from build123d import *

# Parameters (mm, degrees)
F1_DEPTH = 127
F3_DEPTH = 1.00176


with BuildPart() as f1:
    # F0 (on Front) → F1 (new body, symmetric)
    with BuildSketch(Plane.XZ):
        with BuildLine():
            ThreePointArc((-13.5001, 1.99898), (-12.9146123135, 0.5854876865), (-11.50112, 0))
            Line((-11.50112, 0), (11.50112, 0))
            ThreePointArc((11.50112, 0), (12.9146123135, 0.5854876865), (13.5001, 1.99898))
            Line((13.5001, 1.99898), (13.5001, 5.4991))
            ThreePointArc((13.5001, 5.4991), (13.7932158177, 6.2067441823), (14.50086, 6.49986))
            Line((14.50086, 6.49986), (18.3281093243, 6.49986))
            Line((18.3281093243, 6.49986), (18.3281093243, 7.50062))
            Line((18.3281093243, 7.50062), (14.5161, 7.50062))
            ThreePointArc((14.5161, 7.50062), (13.1026076865, 6.9151323135), (12.51712, 5.50164))
            Line((12.51712, 5.50164), (12.51712, 2.00152))
            ThreePointArc((12.51712, 2.00152), (12.2240041823, 1.2938758177), (11.51636, 1.00076))
            Line((11.51636, 1.00076), (-11.48334, 1.00076))
            ThreePointArc((-11.48334, 1.00076), (-12.1909841823, 1.2938758177), (-12.4841, 2.00152))
            Line((-12.4841, 2.00152), (-12.4841, 5.50164))
            ThreePointArc((-12.4841, 5.50164), (-13.0695876865, 6.9151323135), (-14.48308, 7.50062))
            Line((-14.48308, 7.50062), (-16.6730906757, 7.50062))
            Line((-16.6730906757, 7.50062), (-16.6730906757, 6.49986))
            Line((-16.6730906757, 6.49986), (-14.50086, 6.49986))
            ThreePointArc((-14.50086, 6.49986), (-13.7932158177, 6.2067441823), (-13.5001, 5.4991))
            Line((-13.5001, 5.4991), (-13.5001, 1.99898))
        make_face()
    extrude(amount=F1_DEPTH, both=True)

    # F2 (on face) → F3 (cut, through all)
    with BuildSketch(Plane.XY.offset(1.00076)):
        with BuildLine():
            ThreePointArc((2.59969, 9.89965), (0, 12.49934), (-2.59969, 9.89965))
            Line((-2.59969, 9.89965), (-2.59969, -9.89965))
            ThreePointArc((-2.59969, -9.89965), (0, -12.49934), (2.59969, -9.89965))
            Line((2.59969, -9.89965), (2.59969, 9.89965))
        make_face()
        with BuildLine():
            ThreePointArc((-2.59969, 26.09977), (0, 23.50008), (2.59969, 26.09977))
            Line((2.59969, 26.09977), (2.59969, 45.89907))
            ThreePointArc((2.59969, 45.89907), (0, 48.49876), (-2.59969, 45.89907))
            Line((-2.59969, 45.89907), (-2.59969, 26.09977))
        make_face()
        with BuildLine():
            ThreePointArc((-2.59969, 62.09919), (0, 59.4995), (2.59969, 62.09919))
            Line((2.59969, 62.09919), (2.59969, 81.89849))
            ThreePointArc((2.59969, 81.89849), (0, 84.49818), (-2.59969, 81.89849))
            Line((-2.59969, 81.89849), (-2.59969, 62.09919))
        make_face()
        with BuildLine():
            ThreePointArc((-2.59969, 98.09861), (0, 95.49892), (2.59969, 98.09861))
            Line((2.59969, 98.09861), (2.59969, 117.89791))
            ThreePointArc((2.59969, 117.89791), (0, 120.4976), (-2.59969, 117.89791))
            Line((-2.59969, 117.89791), (-2.59969, 98.09861))
        make_face()
        with BuildLine():
            ThreePointArc((-2.59969, -45.89907), (0, -48.49876), (2.59969, -45.89907))
            Line((2.59969, -45.89907), (2.59969, -26.09977))
            ThreePointArc((2.59969, -26.09977), (0, -23.50008), (-2.59969, -26.09977))
            Line((-2.59969, -26.09977), (-2.59969, -45.89907))
        make_face()
        with BuildLine():
            ThreePointArc((-2.59969, -81.89849), (0, -84.49818), (2.59969, -81.89849))
            Line((2.59969, -81.89849), (2.59969, -62.09919))
            ThreePointArc((2.59969, -62.09919), (0, -59.4995), (-2.59969, -62.09919))
            Line((-2.59969, -62.09919), (-2.59969, -81.89849))
        make_face()
        with BuildLine():
            ThreePointArc((-2.59969, -117.89791), (0, -120.4976), (2.59969, -117.89791))
            Line((2.59969, -117.89791), (2.59969, -98.09861))
            ThreePointArc((2.59969, -98.09861), (0, -95.49892), (-2.59969, -98.09861))
            Line((-2.59969, -98.09861), (-2.59969, -117.89791))
        make_face()
    extrude(amount=-F3_DEPTH, mode=Mode.SUBTRACT)


solid = f1.part
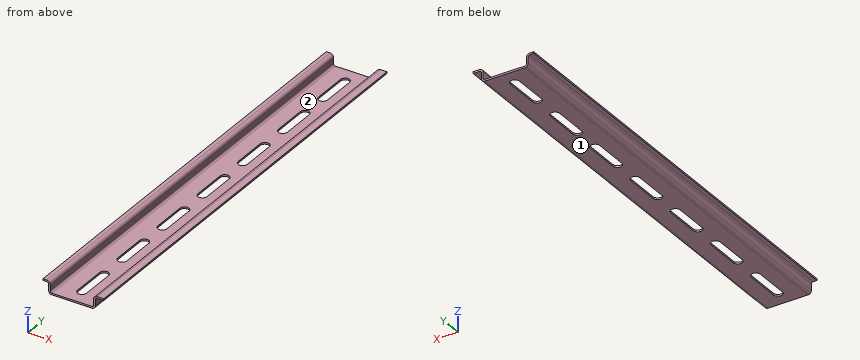
Source: CAD feature listing. Evaluate the final solid. Frame: model axes, mm. Face numbers are marked on the shaded views. Coordinates: 2 decimals unless noted, no trailing zeros. Order: outer loops, then holes, each group sorted by start corner. A loop starts at its lowest first (then second) coordinate and runs counter-clockwise, first axis right, second up.
Item 1: Material intervals for line 1 (X direction, y = -48.5, z = 3); line 2 (Z direction, x = -4.5, y = 21.5); line 3 (Z direction, x = 15, y = -31.5), sorted ascending.
Output values:
line 1: x = -13.5 to -12.48, 12.52 to 13.5
line 2: z = 0 to 1
line 3: z = 6.5 to 7.5
Item 2: Cut plane B-B (z = 3.25). Return loops of the section in (x, y), plus the area to 3 significant figures.
Output values:
outline: (-13.5, -127) - (-12.48, -127) - (-12.48, 127) - (-13.5, 127) - close; (12.52, -127) - (13.5, -127) - (13.5, 127) - (12.52, 127) - close
area: 508 mm2
Item 3: Pull-direction query (X, two-part tool) for the marked faces 1 and 2; classes: pulls with the +X half, pulls with the -X half, needs draft (parallel to the pull), parting line crosses it, or undercut.
Output values:
face 1: needs draft
face 2: undercut
Item 4: Cut plane D-D (y = 89.5). Return loops of the section in (x, z).
Output values:
outline: (-16.67, 6.5) - (-14.5, 6.5) arc R1 cw to (-13.5, 5.5) - (-13.5, 2) arc R2 ccw to (-11.5, 0) - (11.5, 0) arc R2 ccw to (13.5, 2) - (13.5, 5.5) arc R1 cw to (14.5, 6.5) - (18.33, 6.5) - (18.33, 7.5) - (14.52, 7.5) arc R2 ccw to (12.52, 5.5) - (12.52, 2) arc R1 cw to (11.52, 1) - (-11.48, 1) arc R1 cw to (-12.48, 2) - (-12.48, 5.5) arc R2 ccw to (-14.48, 7.5) - (-16.67, 7.5) - close
Item 5: First-contact query: P1, Ø1.1, axis at x = -15, y = -25, coming from the -Z side; P2, Ø1.1, axis at y = 110, z = 0.5, coming from the +X side; P3, Ø0.8, axis at y = -104.5, z = 0.5, coming from the +X side. Flat tips, straight axial feed; report the tip coordinate or a pass-through.
Output values:
P1: stops at z = 6.5
P2: stops at x = 13.26
P3: stops at x = 13.17
Item 6: Cut plane C-C (x = 0). Count the separate pieces of the cut face and the enclosed holes in it, plus the area to 3 significant figures.
Output values:
separate pieces: 8
enclosed holes: 0
area: 79.1 mm2
Item 7: Cut plane A-A (y = -1.5). Return loops of the section in (x, z), plus the area to 3 significant figures.
Output values:
outline: (-16.67, 6.5) - (-14.5, 6.5) arc R1 cw to (-13.5, 5.5) - (-13.5, 2) arc R2 ccw to (-11.5, 0) - (-2.6, 0) - (-2.6, 1) - (-11.48, 1) arc R1 cw to (-12.48, 2) - (-12.48, 5.5) arc R2 ccw to (-14.48, 7.5) - (-16.67, 7.5) - close; (2.6, 0) - (11.5, 0) arc R2 ccw to (13.5, 2) - (13.5, 5.5) arc R1 cw to (14.5, 6.5) - (18.33, 6.5) - (18.33, 7.5) - (14.52, 7.5) arc R2 ccw to (12.52, 5.5) - (12.52, 2) arc R1 cw to (11.52, 1) - (2.6, 1) - close
area: 40.2 mm2
